from build123d import *

# Parameters (mm, degrees)
SKETCH1_W           = 237.6932
SKETCH1_H           = 177.6984
SKETCH1_W_2         = 224.9932
SKETCH1_H_2         = 164.9984
BOSS_EXTRUDE1_DEPTH = 374.65
SKETCH4_W           = 107.442
SKETCH4_H           = 374.65
BOSS_EXTRUDE2_DEPTH = 9.017
SKETCH5_W           = 120.142
SKETCH5_H           = 374.65
BOSS_EXTRUDE3_DEPTH = 4.191
SKETCH7_W           = 9.017
SKETCH7_H           = 107.442
CUT_EXTRUDE1_DEPTH  = 21.59
SKETCH10_W          = 4.191
SKETCH10_H          = 120.142
CUT_EXTRUDE2_DEPTH  = 5.588
FILLET1_R           = 10
FILLET2_R           = 10
FILLET3_R           = 10
FILLET4_R           = 10
FILLET5_R           = 10
FILLET6_R           = 10
FILLET7_R           = 10
SKETCH11_W          = 50.8
SKETCH11_H          = 15.24
BOSS_EXTRUDE4_DEPTH = 19.9898
FILLET10_R          = 10
FILLET11_R          = 10
BOSS_EXTRUDE5_DEPTH = 6.35
FILLET13_R          = 10
SKETCH13_W          = 36.3982
SKETCH13_H          = 16.129
CUT_EXTRUDE4_DEPTH  = 3.175


with BuildPart() as part:
    # Sketch1 → Boss-Extrude1 (new body)
    with BuildSketch(Plane(origin=(0, 0, 0), x_dir=(1, 0, 0), z_dir=(0, 1, 0))):
        with Locations((112.4966, -82.4992)):
            Rectangle(SKETCH1_W, SKETCH1_H)
        with Locations((112.4966, -82.4992)):
            Rectangle(SKETCH1_W_2, SKETCH1_H_2, mode=Mode.SUBTRACT)
    extrude(amount=BOSS_EXTRUDE1_DEPTH)

    # Sketch4 → Boss-Extrude2 (add)
    with BuildSketch(Plane.ZY.offset(-224.9932)):
        with Locations((82.4484, 187.325)):
            Rectangle(SKETCH4_W, SKETCH4_H)
    extrude(amount=BOSS_EXTRUDE2_DEPTH)

    # Sketch5 → Boss-Extrude3 (add)
    with BuildSketch(Plane.ZY.offset(-215.9762)):
        with Locations((82.4484, 187.325)):
            Rectangle(SKETCH5_W, SKETCH5_H)
    extrude(amount=BOSS_EXTRUDE3_DEPTH)

    # Sketch7 → Cut-Extrude1 (cut)
    with BuildSketch(Plane(origin=(0, 374.65, 0), x_dir=(1, 0, 0), z_dir=(0, 1, 0))):
        with Locations((220.4847, -82.4484)):
            Rectangle(SKETCH7_W, SKETCH7_H)
    extrude(amount=-CUT_EXTRUDE1_DEPTH, mode=Mode.SUBTRACT)

    # Sketch10 → Cut-Extrude2 (cut)
    with BuildSketch(Plane(origin=(0, 374.65, 0), x_dir=(1, 0, 0), z_dir=(0, 1, 0))):
        with Locations((213.8807, -82.4484)):
            Rectangle(SKETCH10_W, SKETCH10_H)
    extrude(amount=-CUT_EXTRUDE2_DEPTH, mode=Mode.SUBTRACT)

    # Fillet1
    fillet1_edges = [part.edges().sort_by_distance(p)[0] for p in [
        (231.3432, 187.325, 171.3484),
    ]]
    fillet(fillet1_edges, radius=FILLET1_R)

    # Fillet2
    fillet2_edges = [part.edges().sort_by_distance(p)[0] for p in [
        (224.9932, 187.325, 164.9984),
    ]]
    fillet(fillet2_edges, radius=FILLET2_R)

    # Fillet3
    fillet3_edges = [part.edges().sort_by_distance(p)[0] for p in [
        (224.9932, 187.325, 0),
        (231.3432, 187.325, -6.35),
    ]]
    fillet(fillet3_edges, radius=FILLET3_R)

    # Fillet4
    fillet4_edges = [part.edges().sort_by_distance(p)[0] for p in [
        (0, 187.325, 164.9984),
        (-6.35, 187.325, 171.3484),
    ]]
    fillet(fillet4_edges, radius=FILLET4_R)

    # Fillet5
    fillet5_edges = [part.edges().sort_by_distance(p)[0] for p in [
        (0, 187.325, 0),
        (-6.35, 187.325, -6.35),
    ]]
    fillet(fillet5_edges, radius=FILLET5_R)

    # Fillet6
    fillet6_edges = [part.edges().sort_by_distance(p)[0] for p in [
        (220.4847, 353.06, 28.7274),
        (220.4847, 353.06, 136.1694),
    ]]
    fillet(fillet6_edges, radius=FILLET6_R)

    # Fillet7
    fillet7_edges = [part.edges().sort_by_distance(p)[0] for p in [
        (213.8807, 369.062, 22.3774),
        (213.8807, 369.062, 142.5194),
    ]]
    fillet(fillet7_edges, radius=FILLET7_R)

    # Sketch11 → Boss-Extrude4 (add)
    with BuildSketch(Plane.ZY.offset(-211.7852)):
        with Locations((82.4484, 7.62)):
            Rectangle(SKETCH11_W, SKETCH11_H)
    extrude(amount=BOSS_EXTRUDE4_DEPTH)

    # Fillet10
    fillet10_edges = [part.edges().sort_by_distance(p)[0] for p in [
        (191.7954, 7.62, 57.0484),
        (191.7954, 7.62, 107.8484),
    ]]
    fillet(fillet10_edges, radius=FILLET10_R)

    # Fillet11
    fillet11_edges = [part.edges().sort_by_distance(p)[0] for p in [
        (191.7954, 15.24, 82.4484),
        (206.7903, 15.24, 57.0484),
        (206.7903, 15.24, 107.8484),
        (194.724332188, 15.24, 59.977332188),
        (194.724332188, 15.24, 104.919467812),
    ]]
    fillet(fillet11_edges, radius=FILLET11_R)

    # Sketch12 → Boss-Extrude5 (add)
    with BuildSketch(Plane.XZ):
        with BuildLine():
            Line((231.3432, 161.3484), (231.3432, 3.65))
            ThreePointArc((231.3432, 3.65), (228.414267812, -3.421067812), (221.3432, -6.35))
            Line((221.3432, -6.35), (3.65, -6.35))
            ThreePointArc((3.65, -6.35), (-3.421067812, -3.421067812), (-6.35, 3.65))
            Line((-6.35, 3.65), (-6.35, 161.3484))
            ThreePointArc((-6.35, 161.3484), (-3.421067812, 168.419467812), (3.65, 171.3484))
            Line((3.65, 171.3484), (221.3432, 171.3484))
            ThreePointArc((221.3432, 171.3484), (228.414267812, 168.419467812), (231.3432, 161.3484))
        make_face()
    extrude(amount=BOSS_EXTRUDE5_DEPTH)

    # Fillet13
    fillet13_edges = [part.edges().sort_by_distance(p)[0] for p in [
        (224.9932, 0, 19.3637),
        (222.064267812, 0, 2.928932188),
        (112.4966, 0, 0),
        (2.928932188, 0, 2.928932188),
        (224.9932, 0, 145.5839),
        (222.064267812, 0, 162.069467812),
        (112.4966, 0, 164.9984),
        (2.928932188, 0, 162.069467812),
        (0, 0, 82.4992),
    ]]
    fillet(fillet13_edges, radius=FILLET13_R)

    # Sketch13 → Cut-Extrude4 (cut)
    with BuildSketch(Plane(origin=(0, 0, 0), x_dir=(0, 0, -1), z_dir=(1, 0, 0))):
        with Locations((-82.5551, 346.9767)):
            Rectangle(SKETCH13_W, SKETCH13_H)
    extrude(amount=-CUT_EXTRUDE4_DEPTH, mode=Mode.SUBTRACT)


solid = part.part
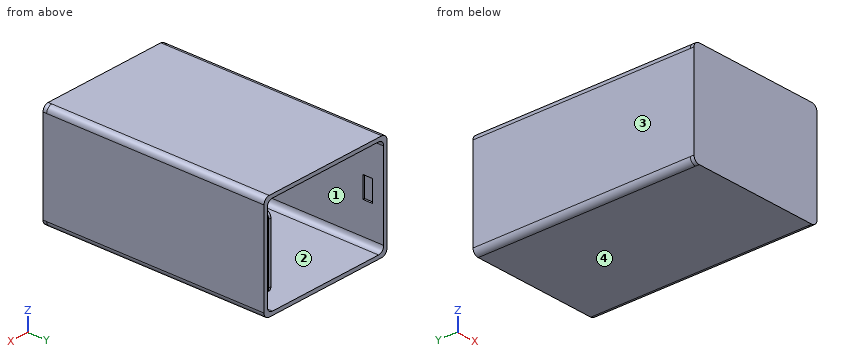
Model file for the job. Use its own axes, mm. Face numbers are marked on the shaded views. Round coordinates to 2 decimals unless told otherwise and drop trailing zeros. Loops run counter-clockwise (first coordinate to the right, second up) from the corner with the lowest first, then second, coordinate; pieces in that order, holes last. Notation, with made-up numbers: (4.25, -19) -> (47.25, -19) arc R25 ccw to (47.25, -5) -> close; hole circle Ø5 at (-40, 50.5). An arc over 180 degrees is marked (long way). Answer as CSV lines item,"result". Start each with the question number.
1) Probe line 1 along X through (y, z) = (214, 27); line 2 along Z through (x, y) = (34.5, 234.5). List the from-to ranges inside material, lowest first.
2) Slice it at A-A (y = 203). List the corners of the cut face in (x, z), plus the area to 3 significant figures.
3) Slice it at B-B (z = 76). List the corners of the cut face in (x, y) (3 decimals).
4) Slice it at D-D (z = 44). List the corners of the cut face in (x, y).
5) Slice it at C-C (x = 108.5). List the corners of the cut face in (y, z), plus the area to 3 significant figures.
6) Pin check, flat tips, straight feed: P1, Ø4, axis at x = 207.5, z = 83.5, coming from the +Y side; P2, Ø8, axis at x = 209, z = 83.5, coming from the +Y side; P3, Ø1, axis at x = 77, z = 12, coming from the +Y side. Stop position of each tip, or through.
7) Mould opens along X. For the marked faces 1, 2, 3 and 4 say: +X half, -X half, draft (parallel to the pull), parting line (faces both ways), or undercut.
Filled in:
1,line 1,"x = -6.35 to 0, 211.79 to 215.98, 224.99 to 231.34"
1,line 2,"z = -6.35 to 0, 165 to 171.35"
2,outline,"(-6.35, 3.65) arc R10 ccw to (3.65, -6.35) -> (221.34, -6.35) arc R10 ccw to (231.34, 3.65) -> (231.34, 161.35) arc R10 ccw to (221.34, 171.35) -> (3.65, 171.35) arc R10 ccw to (-6.35, 161.35) -> close; hole (0, 10) arc R10 ccw to (10, 0) -> (214.99, 0) arc R10 ccw to (224.99, 10) -> (224.99, 28.73) -> (215.98, 28.73) -> (215.98, 22.38) -> (211.79, 22.38) -> (211.79, 142.52) -> (215.98, 142.52) -> (215.98, 136.17) -> (224.99, 136.17) -> (224.99, 155) arc R10 ccw to (214.99, 165) -> (10, 165) arc R10 ccw to (0, 155) -> close"
2,area,"6,590 mm2"
3,outline,"(-6.35, -6.35) -> (231.343, -6.35) -> (231.343, 374.65) -> (224.993, 374.65) -> (224.993, 353.06) -> (215.976, 353.06) -> (215.976, 369.062) -> (211.785, 369.062) -> (211.785, 15.24) -> (201.795, 15.24) arc R10 ccw to (191.795, 5.24) -> (191.795, 0) -> (10, 0) arc R10 cw to (0, 10) -> (0, 338.912) -> (-3.175, 338.912) -> (-3.175, 355.041) -> (0, 355.041) -> (0, 374.65) -> (-6.35, 374.65) -> close"
4,outline,"(-6.35, -6.35) -> (231.34, -6.35) -> (231.34, 374.65) -> (224.99, 374.65) -> (224.99, 353.06) -> (215.98, 353.06) -> (215.98, 369.06) -> (211.79, 369.06) -> (211.79, 0) -> (10, 0) arc R10 cw to (0, 10) -> (0, 374.65) -> (-6.35, 374.65) -> close"
5,outline,"(-6.35, -6.35) -> (374.65, -6.35) -> (374.65, 0) -> (10, 0) arc R10 cw to (0, 10) -> (0, 155) arc R10 cw to (10, 165) -> (374.65, 165) -> (374.65, 171.35) -> (-6.35, 171.35) -> close"
5,area,"5,930 mm2"
6,P1,"stops at y = 15.24"
6,P2,"stops at y = 369.06"
6,P3,"stops at y = 0"
7,face 1,"undercut"
7,face 2,"undercut"
7,face 3,"-X half"
7,face 4,"draft"
